CAD build for the part. Positions are in the model's coordinates, mm. A direction names the side the tool comes from. Coordinates: 2 decimals unless noted, no trailing zeros. Loops run counter-clockwise (first coordinate to the right, second up) from the corner with the lowest first, then second, coordinate; pieces in that order, holes last. Notation, with made-up numbers: (56.5, 47) -> (67.5, 47) arc R35 ccw to (67.5, 83) -> close; hole circle Ø1 at (-4.5, 32.25). An arc over 180 degrees is marked (long way). Return JSON: item names as keys, results as strings. Group by question number.
(1) Saw through at A-A on y = 8. Write the cut outline in (x, z).
(2) Saw through at B-B on z = 2. Write the cut outline in (x, y).
(3) Saw through at D-D on x = -4. Write the cut outline in (y, z).
(4) Mould opens along Y. For faces 1 (the face through (-53.63, -9.25, 7.89)), 2 (the face through (-49.897, 11, 8)), 3 (the face through (11.872, 17.656, 8.901)), 4 (the face through (15.37, 18.85, 8.53)) say: pulls with the +Y half, pulls with the -Y half, needs draft (parallel to the pull), parting line crosses it, or undercut.
(5) Flat gauge pins, fed straight in: pin 1 Ø7.5 at (x, z) = (-11.19, 8) entering from +Y; pin 2 Ø1.5 at (x, z) = (-52.5, 8.5) entering from +Y; pin 3 Ø2.5 at (y, z) = (20.52, 8) entering from -X. Where does each tip first touch, or does it go through?
(6) Tool access for faces 5 (the face through (12.379, 19, 8)), 6 (the face through (-53.376, 21.531, 9.106)), 7 (the face through (-19, -5.483, 8)), 8 (the face through (14.379, 19, 8)), 9 (the face through (-52, 27.141, 8)): list every direction of +Z, -Z, +X, -X, +Y, -Y with a clear straight run to the whole face (end or side of a thin tool).
(7) Probe L1, parallel to X at y = -2.5, z = 11.25; L2, parallel to Y at x = -45.5, z = 5.75; L3, parallel to X at y = -8.5, z = 8. List the from-to ranges inside material, lowest first.
(8) Saw through at C-C on z = 8. Give the number of separate pieces and of enclosed holes in the cut face, then the cut area to 3 significant figures.
```python
from build123d import *

# Parameters (mm, degrees)
BOSS_EXTRUDE1_DEPTH = 16
SKETCH2_R           = 3.25
CUT_EXTRUDE1_DEPTH  = 20
FILLET1_R           = 1
CHAMFER1_SIZE       = 2
SKETCH3_R           = 1.75
CUT_EXTRUDE2_DEPTH  = 20
SKETCH4_R           = 3
CUT_EXTRUDE3_DEPTH  = 3
BOSS_EXTRUDE2_START = 2
SKETCH5_R           = 3
BOSS_EXTRUDE2_DEPTH = 2
SKETCH6_R           = 1
CUT_EXTRUDE4_DEPTH  = 2
SKETCH7_W           = 16
SKETCH7_H           = 5
BOSS_EXTRUDE3_DEPTH = 37
SKETCH8_W           = 5
SKETCH8_H           = 16
BOSS_EXTRUDE4_DEPTH = 37
CUT_EXTRUDE5_START  = -87
SKETCH9_R           = 1
CUT_EXTRUDE5_DEPTH  = 87
SKETCH10_R          = 3.5
CUT_EXTRUDE6_DEPTH  = 2
SKETCH11_R          = 1.5
CUT_EXTRUDE7_DEPTH  = 12
CHAMFER2_SIZE       = 2.5
FILLET2_R           = 1
SKETCH12_W          = 16
SKETCH12_H          = 4.376308933
CUT_EXTRUDE8_DEPTH  = 12


with BuildPart() as part:
    # Sketch1 → Boss-Extrude1 (new body)
    with BuildSketch(Plane.XY):
        Polygon((16.379310345, 29.517241379), (11.379310345, 29.517241379), (11.379310345, -5.482758621), (-17.896551724, -5.482758621), (-17.896551724, -10.482758621), (16.379310345, -10.482758621), align=None)
    extrude(amount=BOSS_EXTRUDE1_DEPTH)

    # Sketch2 → Cut-Extrude1 (cut)
    with BuildSketch(Plane(origin=(0, -5.482758621, 0), x_dir=(1, 0, 0), z_dir=(0, 1, 0))):
        with Locations(Location((-11.192164188, -8, 0), (0, 0, 270))):
            Circle(SKETCH2_R)
    extrude(amount=-CUT_EXTRUDE1_DEPTH, mode=Mode.SUBTRACT)

    # Fillet1
    fillet1_edges = [part.edges().sort_by_distance(p)[0] for p in [
        (11.379310345, -5.482758621, 8),
    ]]
    fillet(fillet1_edges, radius=FILLET1_R)

    # Chamfer1
    chamfer1_edges = [part.edges().sort_by_distance(p)[0] for p in [
        (16.379310345, -10.482758621, 8),
    ]]
    chamfer(chamfer1_edges, length=CHAMFER1_SIZE)

    # Sketch3 → Cut-Extrude2 (cut)
    with BuildSketch(Plane.ZY.offset(-11.379310345)):
        with Locations(Location((8, 20.517241379, 0), (0, 0, 270))):
            Circle(SKETCH3_R)
    extrude(amount=-CUT_EXTRUDE2_DEPTH, mode=Mode.SUBTRACT)

    # Sketch4 → Cut-Extrude3 (cut)
    with BuildSketch(Plane.ZY.offset(-11.379310345)):
        with Locations(Location((8, 20.517241379, 0), (0, 0, 270))):
            Circle(SKETCH4_R)
    extrude(amount=-CUT_EXTRUDE3_DEPTH, mode=Mode.SUBTRACT)

    # Sketch5 → Boss-Extrude2 (add)
    with BuildSketch(Plane.ZY.offset(-14.379310345).offset(BOSS_EXTRUDE2_START)):
        with Locations(Location((8, 20.517241379, 0), (0, 0, 270))):
            Circle(SKETCH5_R)
    extrude(amount=-BOSS_EXTRUDE2_DEPTH)

    # Sketch6 → Cut-Extrude4 (cut)
    with BuildSketch(Plane.ZY.offset(-12.379310345)):
        with Locations(Location((8, 20.517241379, 0), (0, 0, 270))):
            Circle(SKETCH6_R)
    extrude(amount=-CUT_EXTRUDE4_DEPTH, mode=Mode.SUBTRACT)

    # Sketch7 → Boss-Extrude3 (add)
    with BuildSketch(Plane.ZY.offset(17.896551724)):
        with Locations((8, -7.982758621)):
            Rectangle(SKETCH7_W, SKETCH7_H)
    extrude(amount=BOSS_EXTRUDE3_DEPTH)

    # Sketch8 → Boss-Extrude4 (add)
    with BuildSketch(Plane(origin=(0, -5.482758621, 0), x_dir=(1, 0, 0), z_dir=(0, 1, 0))):
        with Locations((-52.396551724, -8)):
            Rectangle(SKETCH8_W, SKETCH8_H)
    extrude(amount=BOSS_EXTRUDE4_DEPTH)

    # Sketch9 → Cut-Extrude5 (cut)
    with BuildSketch(Plane(origin=(14.379310345, 0, 0), x_dir=(0, 0, -1), z_dir=(1, 0, 0)).offset(CUT_EXTRUDE5_START)):
        with Locations(Location((-8, 20.517241379, 0), (0, 0, 270))):
            Circle(SKETCH9_R)
    extrude(amount=CUT_EXTRUDE5_DEPTH, mode=Mode.SUBTRACT)

    # Sketch10 → Cut-Extrude6 (cut)
    with BuildSketch(Plane(origin=(-49.896551724, 0, 0), x_dir=(0, 0, -1), z_dir=(1, 0, 0))):
        with Locations((-8, 20.517241379)):
            Circle(SKETCH10_R)
    extrude(amount=-CUT_EXTRUDE6_DEPTH, mode=Mode.SUBTRACT)

    # Sketch11 → Cut-Extrude7 (cut)
    with BuildSketch(Plane(origin=(-51.896551724, 0, 0), x_dir=(0, 0, -1), z_dir=(1, 0, 0))):
        with Locations((-8, 20.517241379)):
            Circle(SKETCH11_R)
    extrude(amount=-CUT_EXTRUDE7_DEPTH, mode=Mode.SUBTRACT)

    # Chamfer2
    chamfer2_edges = [part.edges().sort_by_distance(p)[0] for p in [
        (-54.896551724, -10.482758621, 8),
    ]]
    chamfer(chamfer2_edges, length=CHAMFER2_SIZE)

    # Fillet2
    fillet2_edges = [part.edges().sort_by_distance(p)[0] for p in [
        (-49.896551724, -5.482758621, 8),
    ]]
    fillet(fillet2_edges, radius=FILLET2_R)

    # Sketch12 → Cut-Extrude8 (cut)
    with BuildSketch(Plane(origin=(-49.896551724, 0, 0), x_dir=(0, 0, -1), z_dir=(1, 0, 0))):
        with Locations((-8, 29.329086913)):
            Rectangle(SKETCH12_W, SKETCH12_H)
    extrude(amount=-CUT_EXTRUDE8_DEPTH, mode=Mode.SUBTRACT)


solid = part.part
```
Geometry results:
{
 "1": {"outline": "(-54.9, 0) -> (-49.9, 0) -> (-49.9, 16) -> (-54.9, 16) -> close; (11.38, 0) -> (16.38, 0) -> (16.38, 16) -> (11.38, 16) -> close"},
 "2": {"outline": "(-54.9, -7.98) -> (-52.4, -10.48) -> (14.38, -10.48) -> (16.38, -8.48) -> (16.38, 29.52) -> (11.38, 29.52) -> (11.38, -4.48) arc R1 cw to (10.38, -5.48) -> (-48.9, -5.48) arc R1 cw to (-49.9, -4.48) -> (-49.9, 27.14) -> (-54.9, 27.14) -> close"},
 "3": {"outline": "(-10.48, 0) -> (-5.48, 0) -> (-5.48, 16) -> (-10.48, 16) -> close"},
 "4": {"face 1": "pulls with the -Y half", "face 2": "needs draft", "face 3": "undercut", "face 4": "undercut"},
 "5": {"pin 1": "y = -5.48", "pin 2": "y = 27.14", "pin 3": "x = 12.38"},
 "6": {"face 5": "none", "face 6": "-X", "face 7": "+Z, -Z, +Y", "face 8": "+X", "face 9": "+Z, -Z, -X, +Y"},
 "7": {"L1": "-54.9 to -49.9, 11.38 to 16.38", "L2": "-10.48 to -5.48", "L3": "-54.38 to -14.44, -7.94 to 16.36"},
 "8": {"separate pieces": "4", "enclosed holes": "0", "area": "617 mm²"}
}
